from build123d import *

# Parameters (mm, degrees)
SKETCH1_W                    = 24
SKETCH1_H                    = 40
BOSS_EXTRUDE1_DEPTH          = 62
SKETCH2_R                    = 16.2
CUT_EXTRUDE1_DEPTH           = 5
SKETCH3_R                    = 7.7
CUT_EXTRUDE2_DEPTH           = 25
SKETCH4_R                    = 2.1
CUT_EXTRUDE3_DEPTH           = 6
CHAMFER1_SIZE                = 1
CIRPATTERN1_COUNT            = 4
CHAMFER1_OF_CIRPATTERN1_SIZE = 1
SKETCH5_R                    = 11.1
CUT_EXTRUDE4_DEPTH           = 8
CUT_EXTRUDE5_START           = -10.02
SKETCH6_R                    = 5.25
CUT_EXTRUDE5_DEPTH           = 10.02
SKETCH7_R                    = 4.2
CUT_EXTRUDE6_DEPTH           = 5.98
SKETCH8_R                    = 2.1
CUT_EXTRUDE7_DEPTH           = 6
CHAMFER2_SIZE                = 1
CIRPATTERN2_COUNT            = 4
CHAMFER2_OF_CIRPATTERN2_SIZE = 1


with BuildPart() as part:
    # Sketch1 → Boss-Extrude1 (new body)
    with BuildSketch(Plane(origin=(0, 0, 0), x_dir=(1, 0, 0), z_dir=(0, 1, 0))):
        Rectangle(SKETCH1_W, SKETCH1_H)
    extrude(amount=BOSS_EXTRUDE1_DEPTH)

    # Sketch2 → Cut-Extrude1 (cut)
    with BuildSketch(Plane.ZY.offset(12)):
        with Locations((0, 20)):
            Circle(SKETCH2_R)
    extrude(amount=-CUT_EXTRUDE1_DEPTH, mode=Mode.SUBTRACT)

    # Sketch3 → Cut-Extrude2 (cut)
    with BuildSketch(Plane.ZY.offset(7)):
        with Locations((0, 20)):
            Circle(SKETCH3_R)
    extrude(amount=-CUT_EXTRUDE2_DEPTH, mode=Mode.SUBTRACT)

    # Sketch4 → Cut-Extrude3 (cut)
    with BuildSketch(Plane.ZY.offset(7)):
        with Locations((0, 31.95)):
            Circle(SKETCH4_R)
    cut_extrude3 = extrude(amount=-CUT_EXTRUDE3_DEPTH, mode=Mode.SUBTRACT)

    # Chamfer1
    chamfer1_edges = [part.edges().sort_by_distance(p)[0] for p in [
        (-7, 31.95, -2.1),
    ]]
    chamfer(chamfer1_edges, length=CHAMFER1_SIZE)

    # CirPattern1: Cut-Extrude3 ×4 about axis
    cirpattern1_axis = Axis((0, 20, 0), (1, 0, 0))
    for i in range(1, CIRPATTERN1_COUNT):
        add(cut_extrude3.rotate(cirpattern1_axis, i * 360 / CIRPATTERN1_COUNT), mode=Mode.SUBTRACT)

    # Chamfer1 of CirPattern1
    chamfer1_of_cirpattern1_edges = [part.edges().sort_by_distance(p)[0] for p in [
        (-7, 22.1, 11.95),
        (-7, 8.05, 2.1),
        (-7, 17.9, -11.95),
    ]]
    chamfer(chamfer1_of_cirpattern1_edges, length=CHAMFER1_OF_CIRPATTERN1_SIZE)

    # Sketch5 → Cut-Extrude4 (cut)
    with BuildSketch(Plane(origin=(12, 0, 0), x_dir=(0, 0, -1), z_dir=(1, 0, 0))):
        with Locations((0, 46.9)):
            Circle(SKETCH5_R)
    extrude(amount=-CUT_EXTRUDE4_DEPTH, mode=Mode.SUBTRACT)

    # Sketch6 → Cut-Extrude5 (cut)
    with BuildSketch(Plane(origin=(4, 0, 0), x_dir=(0, 0, -1), z_dir=(1, 0, 0)).offset(CUT_EXTRUDE5_START)):
        with Locations((0, 46.9)):
            Circle(SKETCH6_R)
    extrude(amount=CUT_EXTRUDE5_DEPTH, mode=Mode.SUBTRACT)

    # Sketch7 → Cut-Extrude6 (cut)
    with BuildSketch(Plane(origin=(-6.02, 0, 0), x_dir=(0, 0, -1), z_dir=(1, 0, 0))):
        with Locations((0, 46.9)):
            Circle(SKETCH7_R)
    extrude(amount=-CUT_EXTRUDE6_DEPTH, mode=Mode.SUBTRACT)

    # Sketch8 → Cut-Extrude7 (cut)
    with BuildSketch(Plane(origin=(4, 0, 0), x_dir=(0, 0, -1), z_dir=(1, 0, 0))):
        with Locations((0, 54.74525)):
            Circle(SKETCH8_R)
    cut_extrude7 = extrude(amount=-CUT_EXTRUDE7_DEPTH, mode=Mode.SUBTRACT)

    # Chamfer2
    # the kernel refuses this chamfer: 1 mm, written as the material it takes off along each edge
    with BuildSketch(Plane(origin=(4, 54.74525, 0), x_dir=(0, 0, -1), z_dir=(0, -1, 0))) as chamfer2_piece_1:
        Polygon((2.1 + CHAMFER2_SIZE, 0), (2.1, -CHAMFER2_SIZE), (2.1, 0), align=None)
    revolve(axis=Axis((4, 54.74525, 0), (1, 0, 0)), mode=Mode.SUBTRACT)

    # CirPattern2: Cut-Extrude7 ×4 about axis
    cirpattern2_axis = Axis((0, 46.9, 0), (1, 0, 0))
    for i in range(1, CIRPATTERN2_COUNT):
        add(cut_extrude7.rotate(cirpattern2_axis, i * 360 / CIRPATTERN2_COUNT), mode=Mode.SUBTRACT)

    # Chamfer2 of CirPattern2
    # the kernel refuses this chamfer: 1 mm, written as the material it takes off along each edge
    with BuildSketch(Plane(origin=(4, 46.9, 7.84525), x_dir=(0, 1, 0), z_dir=(0, 0, -1))) as chamfer2_of_cirpattern2_piece_1:
        Polygon((2.1 + CHAMFER2_OF_CIRPATTERN2_SIZE, 0), (2.1, -CHAMFER2_OF_CIRPATTERN2_SIZE), (2.1, 0), align=None)
    revolve(axis=Axis((4, 46.9, 7.84525), (1, 0, 0)), mode=Mode.SUBTRACT)
    with BuildSketch(Plane(origin=(4, 39.05475, 0), x_dir=(0, 0, 1), z_dir=(0, 1, 0))) as chamfer2_of_cirpattern2_piece_2:
        Polygon((2.1 + CHAMFER2_OF_CIRPATTERN2_SIZE, 0), (2.1, -CHAMFER2_OF_CIRPATTERN2_SIZE), (2.1, 0), align=None)
    revolve(axis=Axis((4, 39.05475, 0), (1, 0, 0)), mode=Mode.SUBTRACT)
    with BuildSketch(Plane(origin=(4, 46.9, -7.84525), x_dir=(0, -1, 0), z_dir=(0, 0, 1))) as chamfer2_of_cirpattern2_piece_3:
        Polygon((2.1 + CHAMFER2_OF_CIRPATTERN2_SIZE, 0), (2.1, -CHAMFER2_OF_CIRPATTERN2_SIZE), (2.1, 0), align=None)
    revolve(axis=Axis((4, 46.9, -7.84525), (1, 0, 0)), mode=Mode.SUBTRACT)


solid = part.part
CAD build for the part. Positions are in the model's coordinates, mm. A direction names the side the tool comes from. Coordinates: 2 decimals unless noted, no trailing zeros. Write each loop counter-clockwise with the first axis right and the second up, starting at its lowest first coordinate (ties: lowest second). Pieces come first, ordered by that corner, then holes. Notation, with made-up numbers: M 17,73.25 L 75,73.25 A28 ccw 75,101.25 Z; hole C 66.25,-21.75 d5. An arc over 180 degrees is marked long. Answer as a JSON object with one key per item and string values. Group by question number.
1) Saw through at D-D (y = 46.9). Write the cut outline in (x, z).
2) Saw through at B-B (y = 20). Write the cut outline in (x, z), plus the area to 3 significant figures.
3) Wall check: line 1 (Z direction, x = 0.15, y = 46.9); line 2 (Y direction, x = 2.25, z = 0); line 3 (Y direction, x = -5.5, z = -0.5). Give the ranges that are in metal, low to high. Write a range as from..to.
4) Tool access for faces 1 (the face through (-6.02, 51, -2)), 2 (the face through (-1, 32, 0)): list every direction of +Z, -Z, +X, -X, +Y, -Y with a clear straight run to the whole face (end or side of a thin tool).
5) Mould opens along Y. For faces 3 (the face through (0, 31, 20)), 4 (the face through (0.535, 36.973, -0.273)) say: +Y half, -Y half, draft (parallel to the pull), parting line (faces both ways), or undercut.
6) Saw through at A-A (x = -4.5). Write the cut outline in (y, z), plus the area to 3 significant figures.
7) Pin check, flat tips, straight feed: pin 1 Ø12 at (x, z) = (-1, 13) entering from -Y; pin 2 Ø2 at (y, z) = (7.5, 1) entering from -X; pin 3 Ø4.5 at (y, z) = (47, 8) entering from +X; pin 4 Ø2 at (y, z) = (31.5, -0.5) entering from -X. Stop position of each tip, or through.
8) Saw through at C-C (z = -11.95). Write the cut outline in (x, y).
Values follow:
{
 "1": {"outline": "M -12,-20 L 12,-20 L 12,-11.1 L 4,-11.1 L 4,-10.95 L 3,-9.95 L -2,-9.95 L -2,-5.75 L 3,-5.75 L 3.5,-5.25 L -6.02,-5.25 L -6.02,-4.2 L -12,-4.2 Z; M -12,4.2 L -6.02,4.2 L -6.02,5.25 L 3.5,5.25 L 3,5.75 L -2,5.75 L -2,9.95 L 3,9.95 L 4,10.95 L 4,11.1 L 12,11.1 L 12,20 L -12,20 Z"},
 "2": {"outline": "M -12,-20 L 12,-20 L 12,-7.7 L -7,-7.7 L -7,-8.85 L -6,-9.85 L -1,-9.85 L -1,-14.05 L -6,-14.05 L -7,-15.05 L -7,-16.2 L -12,-16.2 Z; M -12,16.2 L -7,16.2 L -7,15.05 L -6,14.05 L -1,14.05 L -1,9.85 L -6,9.85 L -7,8.85 L -7,7.7 L 12,7.7 L 12,20 L -12,20 Z", "area": "453 mm2"},
 "3": {"line 1": "z = -20..-9.95, -5.75..-5.25, 5.25..5.75, 9.95..20", "line 2": "y = 0..12.3, 27.7..36.95, 41.15..41.65, 52.15..52.65, 56.85..62", "line 3": "y = 0..6.01, 10.09..12.32, 27.68..29.91, 33.99..41.67, 52.13..62"},
 "4": {"face 1": "+X", "face 2": "-X"},
 "5": {"face 3": "draft", "face 4": "undercut"},
 "6": {"outline": "M 0,-20 L 62,-20 L 62,20 L 0,20 Z; hole C 8.05,0 d4.2; hole C 20,0 d15.4; hole C 20,-11.95 d4.2; hole C 20,11.95 d4.2; hole C 31.95,0 d4.2; hole C 46.9,0 d10.5", "area": "2,150 mm2"},
 "7": {"pin 1": "stops at y = 0", "pin 2": "stops at x = -6.04", "pin 3": "stops at x = 3.33", "pin 4": "stops at x = -1"},
 "8": {"outline": "M -12,0 L 12,0 L 12,62 L -12,62 L -12,30.94 L -7,30.94 L -7,23.1 L -6,22.1 L -1,22.1 L -1,17.9 L -6,17.9 L -7,16.9 L -7,9.06 L -12,9.06 Z"}
}
